Design review of the part built by this model. Coordinates are the model's own, in mm. Give positions to 0.01 mm unless a question says otherwise; leave off trailing zeros. Use CSV: the item, a comma, the result in double quotes.
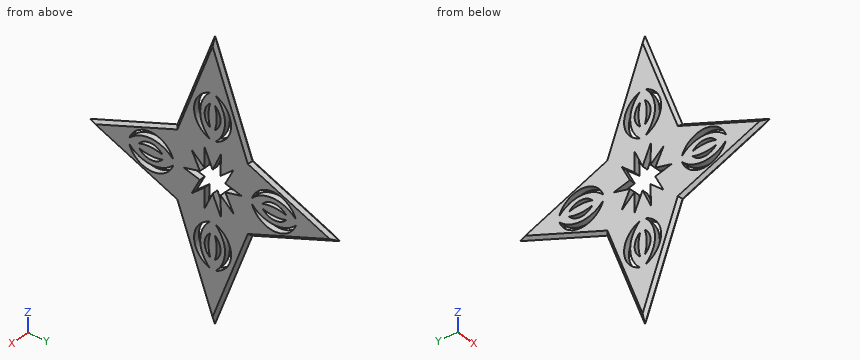
```python
from build123d import *

# Parameters (mm, degrees)
F1_DEPTH = 3
F2_SIZE  = 1.49999
F4_DEPTH = 25
F6_DEPTH = 3.001
F8_COUNT = 4


# Not quite as in the source:
# - a fillet or chamfer is up to 0.001 mm smaller than in the source, because OpenCascade refuses the exact size


with BuildPart() as f1:
    # F0 (on Right) → F1 (new body)
    with BuildSketch(Plane.YZ):
        Polygon((-19.3618498743, -18.3178298175), (0, -70.7087218761), (19.3618498743, -18.3178298175), (64.5395070314, 0), (19.3618498743, 18.3178298175), (0, 70.7087218761), (-19.3618498743, 18.3178298175), (-64.5395070314, 0), align=None)
    extrude(amount=F1_DEPTH)

    # F2 (size 1.5 in the source; OpenCascade refuses exactly that, so slightly less here)
    f2_edges = [f1.edges().sort_by_distance(p)[0] for p in [
        (3, -41.950678, 9.158915),
        (3, -9.680925, 44.513276),
        (0, -9.680925, 44.513276),
        (0, -41.950678, 9.158915),
        (0, -41.950678, -9.158915),
        (3, -41.950678, -9.158915),
        (0, -9.680925, -44.513276),
        (3, -9.680925, -44.513276),
        (3, 9.680925, -44.513276),
        (0, 9.680925, -44.513276),
        (3, 41.950678, -9.158915),
        (0, 41.950678, -9.158915),
        (0, 9.680925, 44.513276),
        (3, 9.680925, 44.513276),
        (3, 41.950678, 9.158915),
        (0, 41.950678, 9.158915),
    ]]
    chamfer(f2_edges, length=F2_SIZE)

    # F3 (on Right) → F4 (cut)
    with BuildSketch(Plane.YZ):
        Polygon((-4.2971530929, -15.4137015343), (0, -5.8852313086), (4.2971530929, -15.4137015343), (4.1103190742, -4.7642351128), (10.8362995088, -10.7428822666), (6.5391454846, -2.1485765465), (14.94661998, 0), (6.5391454846, 2.1485765465), (10.8362995088, 10.7428822666), (4.1103190742, 4.7642351128), (4.2971530929, 15.4137015343), (0, 5.8852313086), (-4.2971530929, 15.4137015343), (-4.1103190742, 4.7642351128), (-10.8362995088, 10.7428822666), (-6.5391454846, 2.1485765465), (-14.94661998, 0), (-6.5391454846, -2.1485765465), (-10.8362995088, -10.7428822666), (-4.1103190742, -4.7642351128), align=None)
    extrude(amount=F4_DEPTH, mode=Mode.SUBTRACT)

    # F5 (on Right) → F6 (cut, through all)
    with BuildSketch(Plane.YZ):
        with BuildLine():
            ThreePointArc((-1.5215650201, -20.3531272709), (-9.5569240867, -31.6740609705), (-1.5215650201, -42.9949946702))
            ThreePointArc((-1.5215650201, -42.9949946702), (-6.4116749119, -31.6740609705), (-1.5215650201, -20.3531272709))
        make_face()
        with BuildLine():
            ThreePointArc((-1.2058431748, -25.8382316679), (-4.0993778142, -31.8839969113), (-1.2058431748, -37.9297621548))
            ThreePointArc((-1.2058431748, -37.9297621548), (-2.1323484034, -31.8839969113), (-1.2058431748, -25.8382316679))
        make_face()
        with BuildLine():
            ThreePointArc((1.5215650201, -20.3531272709), (6.4116749119, -31.6740609705), (1.5215650201, -42.9949946702))
            ThreePointArc((1.5215650201, -42.9949946702), (9.5569240867, -31.6740609705), (1.5215650201, -20.3531272709))
        make_face()
        with BuildLine():
            ThreePointArc((1.2058431748, -25.8382316679), (2.1323484034, -31.8839969113), (1.2058431748, -37.9297621548))
            ThreePointArc((1.2058431748, -37.9297621548), (4.0993778142, -31.8839969113), (1.2058431748, -25.8382316679))
        make_face()
    f6 = extrude(amount=F6_DEPTH, mode=Mode.SUBTRACT)

    # F8: F6 ×4 about axis
    f8_axis = Axis((-24.6906243265, 0, 0), (-1, 0, 0))
    for i in range(1, F8_COUNT):
        add(f6.rotate(f8_axis, i * 360 / F8_COUNT), mode=Mode.SUBTRACT)


solid = f1.part
```
(1) Clearance check with flat-ended pins moving along their axes: pin 1 (1.5 mm diameter, centred on x = 1, z = -48, fed in from +Y); pin 2 (4 mm diameter, centred on y = -40.5, z = -11.5, fed in from -X); pin 3 (1 mm diameter, centred on x = 0.5, z = 26.5, fed in from -Y). State where each tip first meets the part, or that it passes through.
Established:
pin 1,"stops at y = 8.6"
pin 2,"stops at x = 1.12"
pin 3,"stops at y = -15.84"
(2) Take a section at A-A (y = 34). State how many separate pieces and enclosed holes the cut face has, then the cut area to 3 significant figures.
Established:
separate pieces,"5"
enclosed holes,"0"
area,"40.2 mm2"
(3) For line 1 along Z through (x, y) = (1.75, -22); line 2 along Z through (x, y) = (2.4, -37.5); line 3 along Y through (x, z) = (1.8, 21.5), list the stretches that pass through material, from the lowest coordinate up. Write a range as [from, to].
Established:
line 1,"z = [-16.98, -4.65], [-3.04, 3.04], [4.65, 16.98]"
line 2,"z = [-9.99, -8.05], [-5.28, -1.7], [-1.34, 1.34], [1.7, 5.28], [8.05, 9.99]"
line 3,"y = [-17.87, -3.91], [-2.62, 2.62], [3.91, 17.87]"
